Design review of the part built by this model. Coordinates are the model's own, in mm. Face numbers are marked on the shaded views. A direction names the side the tool comes from. Coordinates: 2 decimals unless noted, no trailing zeros. Write each loop counter-clockwise with the first axis right and the second up, starting at its lowest first coordinate (ties: lowest second). Pieces come first, ordered by that corner, then holes. Notation, with made-up numbers: (-12.5, 46.5) - (5.5, 46.5) arc R18 cw to (5.5, 51.5) - close; hole circle Ø4 at (82.5, -3). An arc over 180 degrees is marked (long way). Answer as a JSON object with one key per item and string values.
Autodesk Fusion 360 part; units mm, degrees
sketch "Sketch1" plane through (0, 0, 0) normal (0, 1, 0) x (1, 0, 0)
  line L0 (100, 0) -> (24, 0)
  line L1 (100, 0) -> (176, 0)
  line L2 (176, 0) -> (224, 0) construction
  arc A0 (24, 0) -> (24, 15) centre (24, 7.5) ccw
  arc A1 (176, 15) -> (176, 0) centre (176, 7.5) ccw
  arc A2 (7.5, 15) -> (7.5, 0) centre (7.5, 7.5) ccw
  arc A3 (192.5, 0) -> (192.5, 15) centre (192.5, 7.5) ccw
  arc A4 (7.5, 25) -> (0, 17.5) centre (7.5, 17.5) ccw
  arc A5 (200, 17.5) -> (192.5, 25) centre (192.5, 17.5) ccw
  line L3 (9.5662, 25) -> (12.453, 20)
  line L4 (192.5, 25) -> (190.4338, 25)
  line L5 (190.4338, 25) -> (187.547, 20)
  line L6 (187.547, 20) -> (12.453, 20)
  line L7 (7.5, 25) -> (9.5662, 25)
  line L8 (192.5, 0) -> (7.5, 0)
  line L9 (0, 17.5) -> (0, 7.5)
  line L10 (200, 17.5) -> (200, 7.5)
  line L11 (100, 20) -> (100, 0)
  line L12 (123.25, 15.0004) -> (123.25, 4)
  line L13 (126.75, 15.0004) -> (126.75, 4)
  arc A6 (126.75, 15.0004) -> (123.25, 15.0004) centre (125, 15) ccw
  arc A7 (123.25, 4) -> (126.75, 4) centre (125, 4) ccw
  line L14 (73.25, 15.0004) -> (73.25, 4)
  arc A8 (76.75, 15.0004) -> (73.25, 15.0004) centre (75, 15) ccw
  line L15 (76.75, 15.0004) -> (76.75, 4)
  arc A9 (73.25, 4) -> (76.75, 4) centre (75, 4) ccw
  line L16 (24, 0) -> (12.453, 20)
  line L17 (176, 0) -> (187.547, 20)
  line L18 (176, 15) -> (192.5, 15)
  line L19 (7.5, 15) -> (24, 15)
  point P0 (7.5, 17.5)
  point P1 (192.5, 17.5)
extrude "Extrude1" add sketch "Sketch1" against normal blind 5 makes body 1
extrude "Extrude2" add sketch "Sketch1" along normal blind 5 contours A0 L16 L19 | A2 L8 L16 L19 | A3 L8 L17 L18 | A1 L17 L18 | A2 A4 L3 L7 L9 L16 L19 | A3 A5 L4 L5 L10 L17 L18 bodies 1
extrude "Extrude3" add sketch "Sketch1" along normal blind 10 separate body contours A0 L16 L19 | A2 L8 L16 L19 | A3 L8 L17 L18 | A1 L17 L18 makes body 2 at (18.5, 0, -5) makes body 3 at (187, 0, -5)
extrude "Extrude4" cut sketch "Sketch1" along normal blind 3.5 contours A0 L16 L19 | A1 L17 L18 bodies 2 3
extrude "Extrude5" cut 2 faces at (187, 10, -5) (18.5, 10, -5) along direction (0, -1, 0) blind 1.5 on bodies 2 3 bodies 2 3
extrude "Extrude6" cut 2 faces at (184.3868, 5, -5) (15.6132, 5, -5) along direction (0, -1, 0) blind 5 on bodies 1 bodies 1
combine "Combine1" operation add target body 3 tool bodies 2 1
sketch "Sketch2" plane through (0, 0, 0) normal (0, 1, 0) x (-1, 0, 0)
  arc A0 (-76.75, -15.0004) -> (-73.25, -15.0004) centre (-75, -15) ccw
  line L0 (-76.75, -15.0004) -> (-76.75, -4)
  arc A1 (-73.25, -4) -> (-76.75, -4) centre (-75, -4) ccw
  line L1 (-73.25, -4) -> (-73.25, -15.0004)
  arc A2 (-126.75, -15.0004) -> (-123.25, -15.0004) centre (-125, -15) ccw
  line L2 (-126.75, -15.0004) -> (-126.75, -4)
  arc A3 (-123.25, -4) -> (-126.75, -4) centre (-125, -4) ccw
  line L3 (-123.25, -4) -> (-123.25, -15.0004)
  line L4 (-176, 0) -> (-184.6603, -15)
  line L5 (-184.6603, -15) -> (-192.5, -15)
  arc A4 (-200, -7.5) -> (-192.5, -15) centre (-192.5, -7.5) ccw
  line L6 (-200, -7.5) -> (-200, -17.5)
  arc A5 (-200, -17.5) -> (-192.5, -25) centre (-192.5, -17.5) ccw
  line L7 (-192.5, -25) -> (-190.4338, -25)
  line L8 (-190.4338, -25) -> (-187.547, -20)
  line L9 (-187.547, -20) -> (-12.453, -20)
  line L10 (-12.453, -20) -> (-9.5662, -25)
  line L11 (-9.5662, -25) -> (-7.5, -25)
  arc A6 (-7.5, -25) -> (0, -17.5) centre (-7.5, -17.5) ccw
  line L12 (0, -17.5) -> (0, -7.5)
  arc A7 (-7.5, -15) -> (0, -7.5) centre (-7.5, -7.5) ccw
  line L13 (-7.5, -15) -> (-15.3397, -15)
  line L14 (-15.3397, -15) -> (-24, 0)
  line L15 (-24, 0) -> (-176, 0)
  arc A8 (-76.75, -14.0004) -> (-73.25, -14.0004) centre (-75, -14) ccw
  arc A9 (-73.25, -5) -> (-76.75, -5) centre (-75, -5) ccw
  line L16 (-73.25, -14.0004) -> (-73.25, -5)
  line L17 (-76.75, -5) -> (-76.75, -14.0004)
  line L18 (-100, -20) -> (-100, 0)
  line L19 (-126.75, -4) -> (-126.75, -15.0004)
  line L20 (-123.25, -15.0004) -> (-123.25, -4)
  arc A10 (-126.75, -14.0004) -> (-123.25, -14.0004) centre (-125, -14) ccw
  arc A11 (-123.25, -5) -> (-126.75, -5) centre (-125, -5) ccw
  line L21 (-123.25, -5) -> (-123.25, -14.0004)
  line L22 (-126.75, -14.0004) -> (-126.75, -5)
  point P0 (-125, -4)
  point P1 (-125, -15)
extrude "Extrude7" add sketch "Sketch2" against normal blind 5 contours A0 L0 L1 A8 | L0 A1 L1 A9 | A2 L2 L3 L19 L20 A10 | L2 A3 L3 L19 L20 A11 bodies 3
sketch "Sketch3" plane through (0, 0, 0) normal (0, 1, 0) x (-1, 0, 0)
  arc A0 (-76.75, -14.0004) -> (-73.25, -14.0004) centre (-75, -14) ccw
  line L0 (-76.75, -14.0004) -> (-76.75, -5)
  arc A1 (-73.25, -5) -> (-76.75, -5) centre (-75, -5) ccw
  line L1 (-73.25, -5) -> (-73.25, -14.0004)
  arc A2 (-126.75, -14.0004) -> (-123.25, -14.0004) centre (-125, -14) ccw
  line L2 (-126.75, -14.0004) -> (-126.75, -5)
  arc A3 (-123.25, -5) -> (-126.75, -5) centre (-125, -5) ccw
  line L3 (-123.25, -5) -> (-123.25, -14.0004)
  line L4 (-176, 0) -> (-184.6603, -15)
  line L5 (-184.6603, -15) -> (-192.5, -15)
  arc A4 (-200, -7.5) -> (-192.5, -15) centre (-192.5, -7.5) ccw
  line L6 (-200, -7.5) -> (-200, -17.5)
  arc A5 (-200, -17.5) -> (-192.5, -25) centre (-192.5, -17.5) ccw
  line L7 (-192.5, -25) -> (-190.4338, -25)
  line L8 (-190.4338, -25) -> (-187.547, -20)
  line L9 (-187.547, -20) -> (-12.453, -20)
  line L10 (-12.453, -20) -> (-9.5662, -25)
  line L11 (-9.5662, -25) -> (-7.5, -25)
  arc A6 (-7.5, -25) -> (0, -17.5) centre (-7.5, -17.5) ccw
  line L12 (0, -17.5) -> (0, -7.5)
  arc A7 (-7.5, -15) -> (0, -7.5) centre (-7.5, -7.5) ccw
  line L13 (-7.5, -15) -> (-15.3397, -15)
  line L14 (-15.3397, -15) -> (-24, 0)
  line L15 (-24, 0) -> (-176, 0)
  arc A8 (-7.5, -20) -> (0, -12.5) centre (-7.5, -12.5) ccw
  arc A9 (-200, -12.5) -> (-192.5, -20) centre (-192.5, -12.5) ccw
  line L16 (-192.5, -20) -> (-187.547, -20)
  line L17 (-7.5, -20) -> (-12.453, -20)
extrude "Extrude8" cut sketch "Sketch3" against normal blind 5 contours L6 A5 L7 L8 A9 L16 | L10 L11 A6 L12 A8 L17 bodies 3
fillet "Fillet1" radius 1.6 14 edges at (100, 0, 0) (200, 0, -10) (197.8033, 0, -17.8033) (100, 0, -20) (2.1967, 0, -17.8033) (0, 0, -10) (0, 8.5, -7.5) (15.75, 8.5, -15) (31.5, 8.5, -7.5) (15.75, 8.5, 0) (184.25, 8.5, -15) (200, 8.5, -7.5) (184.25, 8.5, 0) (168.5, 8.5, -7.5) on bodies 3
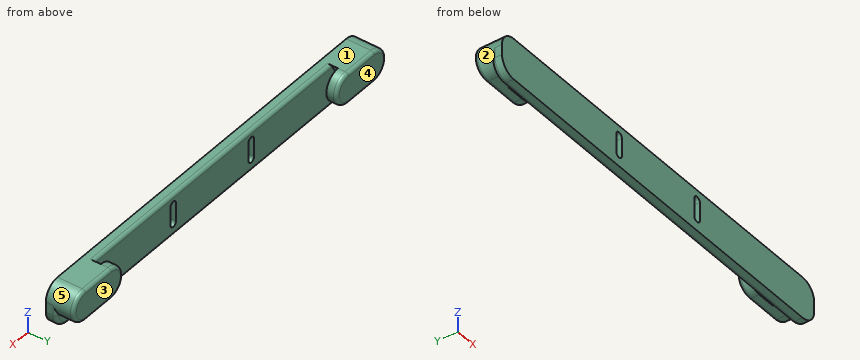
(1) The part is to be moulded in two halves that separate along Z. For the marked faces 1, 2 and 3, say which applies: pulls with the +Z half, pulls with the -Z half, needs draft (parallel to the pull), parting line crosses it, or undercut.
Solved:
{"face 1": "pulls with the +Z half", "face 2": "parting line crosses it", "face 3": "needs draft"}
(2) For pin 1 (1 mm diameter, centred on x = 161, y = 1.5, fed in from -Z); pin 2 (6 mm diameter, centred on y = -2.5, z = -17, fed in from -X); pin 3 (2 mm diameter, centred on x = 185, y = 4.5, fed in from -Z); pin 4 (8.5 mm diameter, centred on x = 91.5, z = -9.5, fed in from +Y), all flat-tipped, find the tip position at first contact; note any pin that passes through.
Solved:
{"pin 1": "passes through", "pin 2": "stops at x = 0.15", "pin 3": "stops at z = -15", "pin 4": "stops at y = 0"}
(3) To check wall thickness, follow line 1 (X direction, y = -3.25, z = -7); line 2 (Y direction, x = 22, z = -13); line 3 (Y direction, x = 61, z = -3.5). State the ranges of each line that lie inside material, in increasing order. Write a range as from..to.
Solved:
{"line 1": "x = 0.02..73.25, 76.75..123.25, 126.75..199.98", "line 2": "y = -5..0, 3.5..8.5", "line 3": "y = -5..0"}
(4) Take a section at B-B, the plane x = 20. Write out the cut boundary in (y, z).
Solved:
{"outline": "(-5, -20) - (-1.6, -20) arc R1.6 ccw to (0, -18.4) - (0, -6.93) - (3.5, -6.93) - (3.5, -15) - (6.9, -15) arc R1.6 ccw to (8.5, -13.4) - (8.5, -1.6) arc R1.6 ccw to (6.9, 0) - (-5, 0) - close"}
(5) Tool access review of the marked faces 4 and 5: name each direction out of +Z, -Z, +X, -X, +Y, -Y from which nothing blocks a thin tool from reaching the whole face with its end or side.
Solved:
{"face 4": "+Z, -Z, +X, -X, +Y", "face 5": "+X, +Y"}
(6) Take a section at A-A, the plane x = 158.5. Write out the cut boundary in (y, z), and give its area (3 significant figures).
Solved:
{"outline": "(-5, -20) - (-1.6, -20) arc R1.6 ccw to (0, -18.4) - (0, -1.6) arc R1.6 ccw to (-1.6, 0) - (-5, 0) - close", "area": "98.9 mm^2"}
